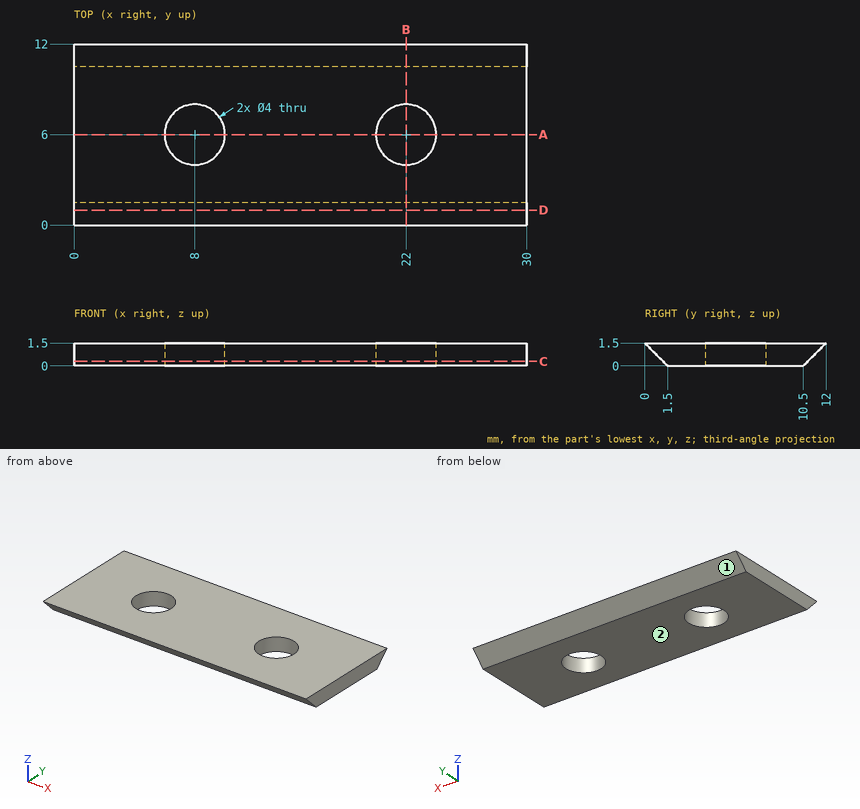
Drawing for the job (mm, zero at the part's lowest x, y, z). Round coordinates to 2 decimals unless told otherwise and drop trailing zeros. Order: outer loops, then holes, each group sorted by start corner. A loop starts at its lowest first (then second) coordinate and runs counter-clockwise, first axis right, second up.
Item 1: Saw through at C-C on z = 0.3. Write the cut outline in (x, y), then the cut area to 3 significant figures.
Item 2: Mould opens along Y. For the marked faces 1 and 2 say: pulls with the +Y half, pulls with the -Y half, needs draft (parallel to the pull), parting line crosses it, or undercut.
Item 3: Saw through at A-A on y = 6. Write the cut outline in (x, z), then the cut area to 3 significant figures.
Item 4: Pin check, flat tip, straight feed: pin 1 (1 mm diameter, centred on x = 7.5, y = 2.5, fed in from -Z). Stop position of the tip, or through.
Item 5: Saw through at B-B on x = 22. Write the cut outline in (y, z), then the cut area to 3 significant figures.
Item 6: Probe line 1 along X through (y, z) = (4.5, 1.1); line 2 along Y through (x, z) = (22, 0.3); line 3 along Y through (x, z) = (8, 1.1). List the from-to ranges inside material, lowest first.
Item 7: Saw through at D-D on y = 1. Write the cut outline in (x, z), then the cut area to 3 significant figures.
Reported:
1. outline: (0, 1.2) - (30, 1.2) - (30, 10.8) - (0, 10.8) - close; hole circle Ø4 at (8, 6); hole circle Ø4 at (22, 6)
1. area: 263 mm2
2. face 1: pulls with the +Y half
2. face 2: needs draft
3. outline: (0, 0) - (6, 0) - (6, 1.5) - (0, 1.5) - close; (10, 0) - (20, 0) - (20, 1.5) - (10, 1.5) - close; (24, 0) - (30, 0) - (30, 1.5) - (24, 1.5) - close
3. area: 33.0 mm2
4. pin 1: stops at z = 0
5. outline: (0, 1.5) - (1.5, 0) - (4, 0) - (4, 1.5) - close; (8, 0) - (10.5, 0) - (12, 1.5) - (8, 1.5) - close
5. area: 9.75 mm2
6. line 1: x = 0 to 6.68, 9.32 to 20.68, 23.32 to 30
6. line 2: y = 1.2 to 4, 8 to 10.8
6. line 3: y = 0.4 to 4, 8 to 11.6
7. outline: (0, 0.5) - (30, 0.5) - (30, 1.5) - (0, 1.5) - close
7. area: 30.0 mm2
